```python
from build123d import *

# Parameters (mm, degrees)
SKETCH1_W           = 120
SKETCH1_H           = 20
BOSS_EXTRUDE1_DEPTH = 60
SKETCH2_R           = 15
BOSS_EXTRUDE2_DEPTH = 30
SKETCH3_R           = 5
CUT_EXTRUDE1_DEPTH  = 76
SKETCH4_R           = 10
CUT_EXTRUDE3_DEPTH  = 30
SKETCH5_W           = 40
SKETCH5_H           = 50
CUT_EXTRUDE5_DEPTH  = 7
SKETCH6_W           = 20
SKETCH6_H           = 8
CUT_EXTRUDE6_DEPTH  = 70
CUT_EXTRUDE7_DEPTH  = 5
CUT_EXTRUDE8_START  = -7
CUT_EXTRUDE8_DEPTH  = 7
CUT_EXTRUDE9_DEPTH  = 24
SKETCH11_W          = 120
SKETCH11_H          = 20
CUT_EXTRUDE10_DEPTH = 4
RIB10_REACH         = 80.102
SKETCH12_WALL_W     = 187.751566924
SKETCH12_WALL_H     = 6
RIB11_REACH         = 80.102
SKETCH13_WALL_W     = 187.751566924
SKETCH13_WALL_H     = 6
FILLET1_R           = 5
SKETCH14_W          = 14
SKETCH14_H          = 10
CUT_EXTRUDE13_DEPTH = 20


with BuildPart() as part:
    # Sketch1 → Boss-Extrude1 (new body)
    with BuildSketch(Plane.XY):
        Rectangle(SKETCH1_W, SKETCH1_H)
    extrude(amount=BOSS_EXTRUDE1_DEPTH)

    # Sketch2 → Boss-Extrude2 (add)
    with BuildSketch(Plane(origin=(0, 10, 0), x_dir=(1, 0, 0), z_dir=(0, 1, 0))):
        with Locations(Location((0, -30, 0), (0, 0, 90))):
            Circle(SKETCH2_R)
    extrude(amount=BOSS_EXTRUDE2_DEPTH)

    # Sketch3 → Cut-Extrude1 (cut)
    with BuildSketch(Plane(origin=(0, 40, 0), x_dir=(1, 0, 0), z_dir=(0, 1, 0))):
        with Locations(Location((0, -30, 0), (0, 0, 270))):
            Circle(SKETCH3_R)
    extrude(amount=-CUT_EXTRUDE1_DEPTH, mode=Mode.SUBTRACT)

    # Sketch4 → Cut-Extrude3 (cut)
    with BuildSketch(Plane(origin=(0, 40, 0), x_dir=(1, 0, 0), z_dir=(0, 1, 0))):
        with Locations(Location((0, -30, 0), (0, 0, 270))):
            Circle(SKETCH4_R)
    extrude(amount=-CUT_EXTRUDE3_DEPTH, mode=Mode.SUBTRACT)

    # Sketch5 → Cut-Extrude5 (cut)
    with BuildSketch(Plane.XZ.offset(10)):
        with Locations((0, 30)):
            Rectangle(SKETCH5_W, SKETCH5_H)
    extrude(amount=-CUT_EXTRUDE5_DEPTH, mode=Mode.SUBTRACT)

    # Sketch6 → Cut-Extrude6 (cut)
    with BuildSketch(Plane.XY.offset(60)):
        with Locations((0, -10)):
            Rectangle(SKETCH6_W, SKETCH6_H)
    extrude(amount=-CUT_EXTRUDE6_DEPTH, mode=Mode.SUBTRACT)

    # Sketch7 → Cut-Extrude7 (cut)
    with BuildSketch(Plane(origin=(0, 10, 0), x_dir=(1, 0, 0), z_dir=(0, 1, 0))):
        with BuildLine():
            Line((-30, -22), (-30, -38))
            ThreePointArc((-30, -38), (-40, -48), (-50, -38))
            Line((-50, -38), (-50, -22))
            ThreePointArc((-50, -22), (-40, -12), (-30, -22))
        make_face()
        with BuildLine():
            Line((50, -22), (50, -38))
            ThreePointArc((50, -38), (40, -48), (30, -38))
            Line((30, -38), (30, -22))
            ThreePointArc((30, -22), (40, -12), (50, -22))
        make_face()
    extrude(amount=-CUT_EXTRUDE7_DEPTH, mode=Mode.SUBTRACT)

    # Sketch9 → Cut-Extrude8 (cut)
    with BuildSketch(Plane.XZ.offset(10).offset(CUT_EXTRUDE8_START)):
        with BuildLine():
            Line((-30, 38), (-30, 22))
            ThreePointArc((-30, 22), (-40, 12), (-50, 22))
            Line((-50, 22), (-50, 38))
            ThreePointArc((-50, 38), (-40, 48), (-30, 38))
        make_face()
        with BuildLine():
            Line((50, 38), (50, 22))
            ThreePointArc((50, 22), (40, 12), (30, 22))
            Line((30, 22), (30, 38))
            ThreePointArc((30, 38), (40, 48), (50, 38))
        make_face()
    extrude(amount=CUT_EXTRUDE8_DEPTH, mode=Mode.SUBTRACT)

    # Sketch10 → Cut-Extrude9 (cut)
    with BuildSketch(Plane(origin=(0, 5, 0), x_dir=(1, 0, 0), z_dir=(0, 1, 0))):
        with BuildLine():
            Line((-45, -38), (-45, -22))
            ThreePointArc((-45, -22), (-40, -17), (-35, -22))
            Line((-35, -22), (-35, -38))
            ThreePointArc((-35, -38), (-40, -43), (-45, -38))
        make_face()
        with BuildLine():
            Line((45, -38), (45, -22))
            ThreePointArc((45, -22), (40, -17), (35, -22))
            Line((35, -22), (35, -38))
            ThreePointArc((35, -38), (40, -43), (45, -38))
        make_face()
    extrude(amount=-CUT_EXTRUDE9_DEPTH, mode=Mode.SUBTRACT)

    # Sketch11 → Cut-Extrude10 (cut)
    with BuildSketch(Plane.XZ.offset(10)):
        with Locations((0, 30)):
            Rectangle(SKETCH11_W, SKETCH11_H)
    extrude(amount=-CUT_EXTRUDE10_DEPTH, mode=Mode.SUBTRACT)

    # Sketch12 wall → Rib10 (add, up to next)
    with BuildSketch(Plane(origin=(-21, 23.5, 30), x_dir=(-0.406138466053, -0.91381154862, 0), z_dir=(0.91381154862, -0.406138466053, 0)), mode=Mode.PRIVATE) as rib10_sk1:
        Rectangle(SKETCH12_WALL_W, SKETCH12_WALL_H)
    rib10_tool1 = extrude(rib10_sk1.sketch, amount=RIB10_REACH, mode=Mode.PRIVATE) - part.part
    add(rib10_tool1.solids().sort_by_distance((-21, 23.5, 30))[0])

    # Sketch13 wall → Rib11 (add, up to next)
    with BuildSketch(Plane(origin=(21, 23.5, 30), x_dir=(0.406138466053, -0.91381154862, 0), z_dir=(0.91381154862, 0.406138466053, 0)), mode=Mode.PRIVATE) as rib11_sk1:
        Rectangle(SKETCH13_WALL_W, SKETCH13_WALL_H)
    rib11_tool1 = extrude(rib11_sk1.sketch, amount=-RIB11_REACH, mode=Mode.PRIVATE) - part.part
    add(rib11_tool1.solids().sort_by_distance((21, 23.5, 30))[0])

    # Fillet1
    fillet1_edges = [part.edges().sort_by_distance(p)[0] for p in [
        (-60, 0, 60),
        (60, 0, 60),
        (-60, 0, 0),
        (60, 0, 0),
    ]]
    fillet(fillet1_edges, radius=FILLET1_R)

    # Sketch14 → Cut-Extrude13 (cut, symmetric)
    with BuildSketch(Plane.XY.offset(30)):
        with Locations((0, 35)):
            Rectangle(SKETCH14_W, SKETCH14_H)
    extrude(amount=CUT_EXTRUDE13_DEPTH, both=True, mode=Mode.SUBTRACT)


solid = part.part
```
Build history of the part. All positions in model axes, mm. A direction names the side the tool comes from. Give positions to 0.01 mm unless a question says otherwise; leave off trailing zeros. Loops run counter-clockwise (first coordinate to the right, second up) from the corner with the lowest first, then second, coordinate; pieces in that order, holes last.
1) Probe line 1 along X through (y, z) = (6.5, 30); line 2 along X through (y, z) = (3, 30); line 3 along Y through (x, z) = (40, 56.5). List the from-to ranges inside material, lowest first.
Values follow:
line 1: x = -60 to -50, -30 to -5, 5 to 30, 50 to 60
line 2: x = -60 to -45, -35 to -5, 5 to 35, 45 to 60
line 3: y = -10 to 10
2) 3-axis set-ups, long thin cutter, end or side, ignore diameter. For faces 4 (the face through (45, 1, 30)), 5 (the face through (40, -6, 12)), 6 (the face through (25, -8, 40)): which of +Z, -Z, +X, -X, +Y, -Y reach the whole face in a straight line?
Values follow:
face 4: +Y, -Y
face 5: -Y
face 6: +X, -X, -Y
3) Band-saw the part on C-C on x = 40. List the corners of the cut face in (y, z).
Values follow:
outline: (-10, 0) - (10, 0) - (10, 12) - (5, 12) - (5, 17) - (-3, 17) - (-3, 12) - (-10, 12) - close; (-10, 48) - (-3, 48) - (-3, 43) - (5, 43) - (5, 48) - (10, 48) - (10, 60) - (-10, 60) - close
4) Band-saw the part on B-B on y = 34.5. List the corners of the cut face in (x, z).
Values follow:
outline: (-16.11, 27) - (-14.7, 27) arc R15 ccw to (-7, 16.73) - (-7, 22.86) arc R10 cw to (-7, 37.14) - (-7, 43.27) arc R15 ccw to (-14.7, 33) - (-16.11, 33) - close; (7, 16.73) arc R15 ccw to (14.7, 27) - (16.11, 27) - (16.11, 33) - (14.7, 33) arc R15 ccw to (7, 43.27) - (7, 37.14) arc R10 cw to (7, 22.86) - close
5) Two-plate mould, pull along Z, no slides. Class faces 1 (the face through (58, 0, 59)), 2 (the face through (-60, 0, 30)), 3 (the face through (40, 8, 48)): released by +Z, released by -Z, zero draft, split by the parting line, or undercut.
Values follow:
face 1: released by +Z
face 2: zero draft
face 3: undercut
6) Drop flat-ended pins along their axis: P1, Ø16, axis at x = 35.5, z = 32.5, coming from the -Y side; P2, Ø4.5, axis at y = -8.5, z = 1.5, coming from the +X side; P3, Ø1.5, axis at x = 9.5, y = 33, coming from the +Z side; P4, Ø3, axis at y = 13, z = 10, coming from the -X side. Give the stop position or say it passes through.
Values follow:
P1: stops at y = -6
P2: stops at x = 59.84
P3: stops at z = 42.18
P4: passes through
7) Band-saw the part on D-D on y = 15. List the corners of the cut face in (x, z), then the cut area to 3 significant figures.
Values follow:
outline: (-24.78, 27) - (-14.7, 27) arc R15 ccw to (14.7, 27) - (24.78, 27) - (24.78, 33) - (14.7, 33) arc R15 ccw to (-14.7, 33) - (-24.78, 33) - close; hole circle Ø20 at (0, 30)
area: 511 mm2
8) Band-saw the part on A-A on x = 0. List the corners of the cut face in (y, z).
Values follow:
outline: (-6, 0) - (10, 0) - (10, 15) - (30, 15) - (30, 20) - (10, 20) - (10, 25) - (-3, 25) - (-3, 5) - (-6, 5) - close; (-6, 55) - (-3, 55) - (-3, 35) - (10, 35) - (10, 40) - (30, 40) - (30, 45) - (10, 45) - (10, 60) - (-6, 60) - close
